Source: three-view drawing plus pictorial views. Frame: mm from the lowest corner of the part. A direction names the side the tool comes from. Coordinates: 2 decimals unless noted, no trailing zeros. Write each loop counter-clockwise with the first axis right and the second up, starting at its lowest first coordinate (ties: lowest second). Pieces come first, ordered by that corner, then holes. Notation, with made-up numbers: (8, 14.5) -> (55, 14.5) arc R25 ccw to (55, 41.5) -> close; hole circle Ø3 at (56.25, 88). An arc over 180 degrees is marked (long way). One line per item, written item: value.
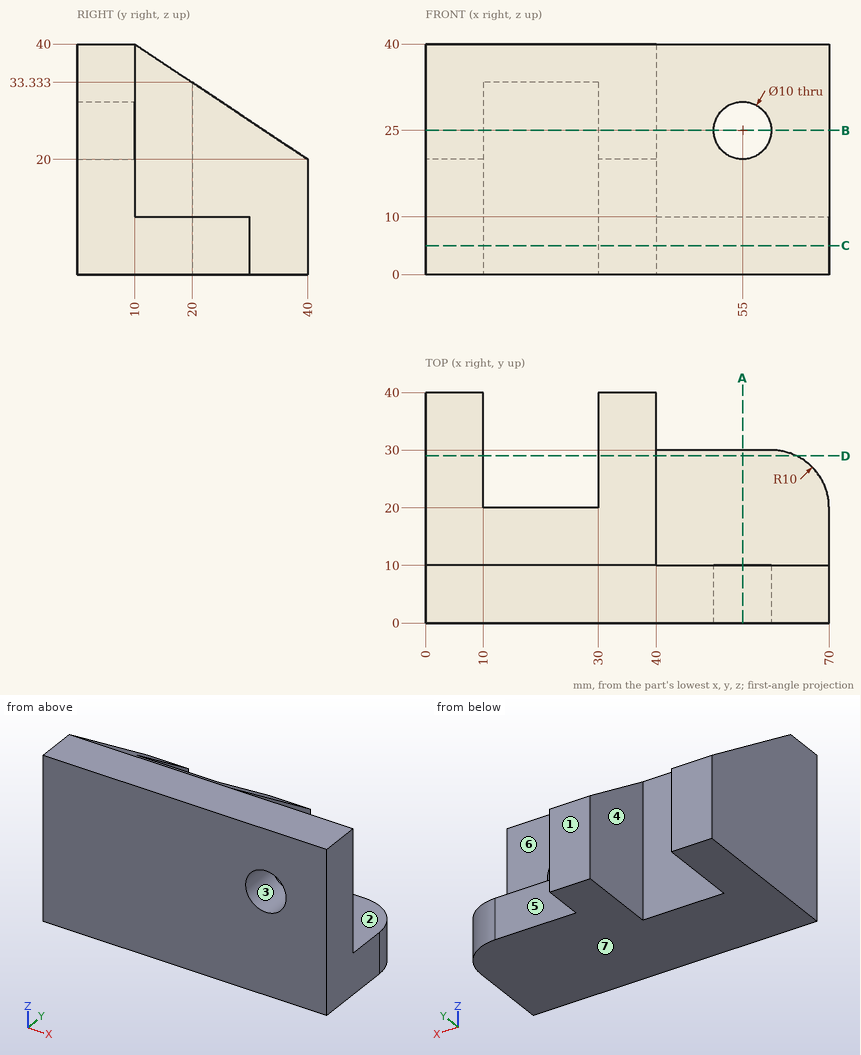
(1) Section C-C (z = 5). Return the cut outline in (x, y), then the cut area to 3 significant figures.
Responses:
outline: (0, 0) -> (70, 0) -> (70, 20) arc R10 ccw to (60, 30) -> (40, 30) -> (40, 40) -> (30, 40) -> (30, 20) -> (10, 20) -> (10, 40) -> (0, 40) -> close
area: 2,080 mm2
(2) Section A-A (x = 55). Return the cut outline in (y, z).
Responses:
outline: (0, 0) -> (30, 0) -> (30, 10) -> (10, 10) -> (10, 20) -> (0, 20) -> close; (0, 30) -> (10, 30) -> (10, 40) -> (0, 40) -> close
(3) Reachability of the marked faces 4, 5, 6 and 7 from +Z, -Z, +X, -X, +Y, -Y: full face, straight path, thin tool, end or side. Return the list, or none.
Responses:
face 4: +Z, -Z, +Y
face 5: +Z, -Z, +X, +Y
face 6: +Z, +X, +Y
face 7: -Z, +X, -X, +Y, -Y
(4) Section D-D (y = 29). Return the cut outline in (x, z).
Responses:
outline: (0, 0) -> (10, 0) -> (10, 27.33) -> (0, 27.33) -> close; (30, 0) -> (64.36, 0) -> (64.36, 10) -> (40, 10) -> (40, 27.33) -> (30, 27.33) -> close
(5) Section B-B (z = 25). Return the cut outline in (x, y), then the cut area to 3 significant figures.
Responses:
outline: (0, 0) -> (50, 0) -> (50, 10) -> (40, 10) -> (40, 32.5) -> (30, 32.5) -> (30, 20) -> (10, 20) -> (10, 32.5) -> (0, 32.5) -> close; (60, 0) -> (70, 0) -> (70, 10) -> (60, 10) -> close
area: 1,250 mm2
(6) Line query: line 1 (X direction, y = 6.75, z = 25); line 2 (Z direction, x = 55, y = 4); line 3 (Y direction, x = 19.5, z = 30). Output: solid intervals per line, ascending. Write a range as [from, to].
Responses:
line 1: x = [0, 50], [60, 70]
line 2: z = [0, 20], [30, 40]
line 3: y = [0, 20]
(7) Pull-direction query (Z, two-part tool) for the marked faces 1, 2 and 3; classes: released by +Z, released by -Z, zero draft, split by the parting line, or undercut.
Responses:
face 1: zero draft
face 2: released by +Z
face 3: undercut
(8) First-contact query: pin 1 (22 mm diameter, centred on y = 32.5, z = 21.5, fed in from +X); pin 2 (6 mm diameter, centred on x = 62.5, y = 24.5, fed in from +Z); pin 3 (16 mm diameter, centred on x = 21.5, z = 10, fed in from +Y). Flat tips, straight axial feed; report the tip coordinate or a pass-through.
Responses:
pin 1: stops at x = 40
pin 2: stops at z = 10
pin 3: stops at y = 20
